Source: CAD feature listing. Evaluate the final solid. Frame: model axes, mm. A direction names the side the tool comes from. Round coordinates to 2 decimals unless told otherwise and drop trailing zeros. Order: outer loops, then holes, each group sorted by start corner. A loop starts at its lowest first (then second) coordinate and runs counter-clockwise, first axis right, second up. Notation, with made-up numbers: (41.5, -10.75) - (50.5, -10.75) arc R14 ccw to (50.5, 4.25) - close; hole circle Ø8 at (-15, 26). An arc over 180 degrees is marked (long way). Use one line per item in the form item = value. Start each with the question number.
Q1. Cut plane D-D, the plane x = 17.5. Return the cut outline in (y, z).
Q2. Ray query, line 1 (Z direction, x = 2.8, y = 12.5); line 2 (Z direction, x = 12.5, y = 1.9) (3 decimals); line 3 (Z direction, x = 2.5, y = 15). Return the intervals inside material, ascending. Write a range as [from, to].
Q3. Cut plane C-C, the plane z = 25. Return the cut outline in (x, y).
Q4. Pin query (flat end, axial travel): pin 1 Ø11.5 at (x, z) = (12.5, 25) entering from +Y; pin 2 Ø1.5 at (x, z) = (17, 34.5) entering from +Y; pin 3 Ø9.5 at (y, z) = (14.5, 29) entering from +X. Return the tip coordinate at first contact, or that it passes through.
Q5. Draft query along X for faces 1 (the flat face through (0, 12, 25)), 2 (the flat face through (4, 7, 0)), 3 (the flat face through (25, 3, 25)), 4 (the cylindrical face through (12.923, 2.958, 37.453)). Return one class per face: released by +X, released by -X, zero draft, split by the parting line, or undercut.
Q6. Cut plane B-B, the plane x = 12.5. Return the cut outline in (y, z) (3 decimals).
Q7. Cut plane A-A, the plane y = 12.5. Return the cut outline in (x, z), and give its area (3 significant figures).
Q8. Set-up query: faces 5 (the flat face through (15.5, 0, 30.9)), 6 (the flat face through (6, 15, 25)). Return all of +Z, -Z, +X, -X, +Y, -Y with unobstructed straight access to the full face (end or side cutting, diameter ignored); none if empty.
Autodesk Inventor part; units mm, degrees
ref_plane "YZ Plane" through (0, 0, 0) normal (1, 0, 0) x (0, 1, 0)
ref_plane "XZ Plane" through (0, 0, 0) normal (0, 1, 0) x (-1, 0, 0)
ref_plane "XY Plane" through (0, 0, 0) normal (0, 0, 1) x (1, 0, 0)
sketch "Sketch1" plane through (0, 0, 0) normal (0, 1, 0) x (-1, 0, 0)
  line L0 (0, 0) -> (0, 50)
  line L1 (0, 50) -> (-25, 50)
  line L2 (-25, 50) -> (-25, 0)
  line L3 (-25, 0) -> (0, 0)
  circle A0 centre (-12.5, 25) radius 6.35
  circle A1 centre (-12.5, 40.675) radius 3.25
  circle A2 centre (-12.5, 9.325) radius 3.25
  dimension "d0" = 50
  dimension "d1" = 25
  dimension "d2" = 12.7
  dimension "d3" = 6.5
  dimension "d4" = 6.5
extrude "Extrusion1" add sketch "Sketch1" along normal blind 6
sketch "Sketch2" plane through (0, 6, 0) normal (0, 1, 0) x (1, 0, 0)
  line L0 (25, 0) -> (0, 0)
  line L1 (0, 0) -> (6, 0)
  line L2 (6, 0) -> (6, -50)
  line L3 (0, -50) -> (25, -50)
  line L4 (0, 0) -> (0, -50)
  line L5 (0, -50) -> (0, 0)
  dimension "d7" = 6
extrude "Extrusion2" add sketch "Sketch2" along normal blind 19
sketch "Sketch3" plane through (6, 6, 50) normal (1, 0, 0) x (0, 0, -1)
  circle A0 centre (16.6667, 6.5) radius 3.25
  circle A1 centre (33.3333, 6.5) radius 3.25
  point P0 (50, -6)
  dimension "d10" = 6.5
  dimension "d11" = 6.5
hole "Hole1" at (6, 12.5, 33.3333) at (6, 12.5, 16.6667) direction (-1, 0, 0) diameter 6.5 depth 111
properties part number "Roter_shaft_support_base"
Completed:
q1.outline = (0, 0) - (6, 0) - (6, 21.09) - (0, 21.09) - close; (0, 28.91) - (6, 28.91) - (6, 50) - (0, 50) - close
q2.line_1 = [0, 13.42], [19.92, 30.08], [36.58, 50]
q2.line_2 = [0, 6.075], [12.575, 18.65], [31.35, 37.425], [43.925, 50]
q2.line_3 = [0, 14.59], [18.74, 31.26], [35.41, 50]
q3.outline = (0, 0) - (6.15, 0) - (6.15, 6) - (6, 6) - (6, 25) - (0, 25) - close; (18.85, 0) - (25, 0) - (25, 6) - (18.85, 6) - close
q4.pin_1 = through
q4.pin_2 = 6
q4.pin_3 = 6
q5.face_1 = released by -X
q5.face_2 = zero draft
q5.face_3 = released by +X
q5.face_4 = undercut
q6.outline = (0, 0) - (6, 0) - (6, 6.075) - (0, 6.075) - close; (0, 12.575) - (6, 12.575) - (6, 18.65) - (0, 18.65) - close; (0, 31.35) - (6, 31.35) - (6, 37.425) - (0, 37.425) - close; (0, 43.925) - (6, 43.925) - (6, 50) - (0, 50) - close
q7.outline = (0, 0) - (6, 0) - (6, 13.42) - (0, 13.42) - close; (0, 19.92) - (6, 19.92) - (6, 30.08) - (0, 30.08) - close; (0, 36.58) - (6, 36.58) - (6, 50) - (0, 50) - close
q7.area = 222 mm2
q8.face_5 = +Z, -Z, +X, -X, -Y
q8.face_6 = +Z, -Z, +X, +Y
